CAD build for the part. Positions are in the model's coordinates, mm. Coordinates: 2 decimals unless noted, no trailing zeros. Order: outer loops, then holes, each group sorted by start corner. A loop starts at its lowest first (then second) coordinate and runs counter-clockwise, first axis right, second up. Notation, with made-up numbers: (66.5, 17) - (99.5, 17) arc R15 cw to (99.5, 27) - close; hole circle Ø3 at (-6.75, -32). An arc over 180 degrees is marked (long way). Use one line per item in the form item = value.
```python
from build123d import *

# Parameters (mm, degrees)
F1_DEPTH = 192
F5_DEPTH = 12.5
F6_R     = 2.05
F7_DEPTH = 200


with BuildPart() as f1:
    # F0 (on Front) → F1 (new body)
    with BuildSketch(Plane.XZ):
        Polygon((0, 12.124355653), (-7, 0), (7, 0), align=None)
    extrude(amount=-F1_DEPTH)

    # F4 (on 3pt) → F5 (cut, symmetric)
    with BuildSketch(Plane(origin=(1.75, 0, 3.0310889132), x_dir=(0.8660254038, 0, -0.5), z_dir=(0.5, 0, 0.8660254038))):
        Polygon((-6.0621778265, 20.5), (-2.5621778265, 17), (-2.5621778265, 174), (-6.0621778265, 171.5), align=None)
    extrude(amount=F5_DEPTH, both=True, mode=Mode.SUBTRACT)

    # F6 (on Front) → F7 (cut)
    with BuildSketch(Plane.XZ):
        with Locations((1.9770526581, 2.9)):
            Circle(F6_R)
    extrude(amount=-F7_DEPTH, mode=Mode.SUBTRACT)


solid = f1.part
```
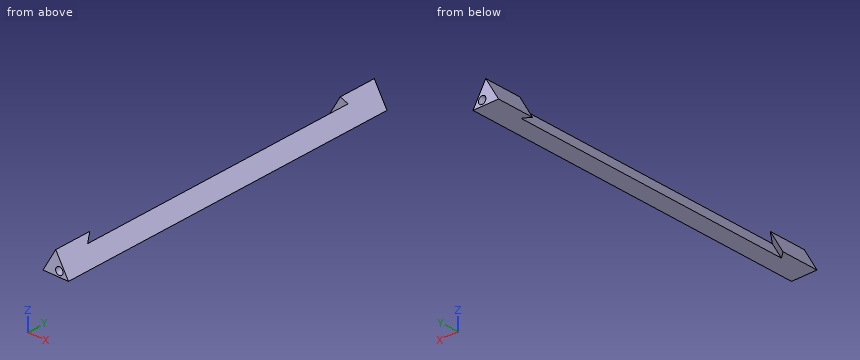
Item 1: Drill centre lines: line 1 (Y direction, x = -3.5, z = 1.5); line 2 (Z direction, x = 2.25, y = 121); line 3 (Y direction, x = -2.75, z = 7.25). Where is each one in solid material? Low to high. Write a range as [from, to].
Derived:
line_1 = [0, 18.22], [173.13, 192]
line_2 = [0, 0.87], [4.93, 8.23]
line_3 = [0, 20.44], [171.54, 192]
Item 2: Cut at B-B, the plane y = 75. Write the cut outline in (x, z), plus the area to 3 significant figures.
Derived:
outline = (-2.96, 0) - (7, 0) - (2.02, 8.62) - close; hole circle Ø4.1 at (1.98, 2.9)
area = 29.7 mm²
Item 3: Cut at A-A, the plane z = 2.9. Write the cut outline in (x, y).
Derived:
outline = (-5.33, 0) - (-0.07, 0) - (-0.07, 192) - (-5.33, 192) - (-5.33, 171.5) - (-1.28, 174) - (-1.28, 17) - (-5.33, 20.5) - close; (4.03, 0) - (5.33, 0) - (5.33, 192) - (4.03, 192) - close
Item 4: Drop flat-ended pins along their axis: pin 1 (2 mm diameter, centred on y = 62.5, z = 2.5, fed in from +X); pin 2 (3 mm diameter, centred on y = 124.5, z = 4.5, fed in from +X); pin 3 (8 mm diameter, centred on x = -4, y = 27, fed in from +Z); pin 4 (1.5 mm diameter, centred on x = -5, y = 152, fed in from +Z). Give the stop position or say it passes through.
Derived:
pin_1 = 6.13
pin_2 = 5.27
pin_3 = 5.12
pin_4 = through
